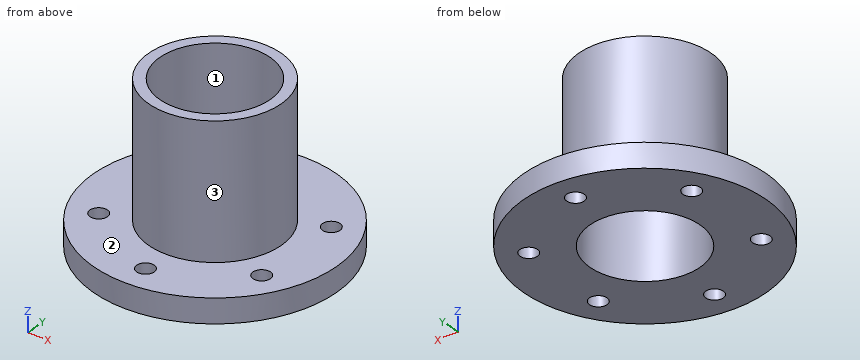
```python
from build123d import *

# Parameters (mm, degrees)
SKETCH1_R               = 110
BOSS_EXTRUDE2_DEPTH     = 22
SKETCH2_R               = 60
BOSS_EXTRUDE3_DEPTH     = 120
CUT_EXTRUDE1_DEPTH      = 211.627633515
CUT_EXTRUDE1_DEPTH_BACK = 211.627633515
SKETCH3_R               = 50
SKETCH4_R               = 8
CUT_EXTRUDE2_DEPTH      = 197.468827044
CIRPATTERN1_COUNT       = 6


with BuildPart() as part:
    # Sketch1 → Boss-Extrude2 (new body)
    with BuildSketch(Plane.XY):
        Circle(SKETCH1_R)
    extrude(amount=BOSS_EXTRUDE2_DEPTH)

    # Sketch2 → Boss-Extrude3 (add)
    with BuildSketch(Plane.XY.offset(22)):
        Circle(SKETCH2_R)
    extrude(amount=BOSS_EXTRUDE3_DEPTH)

    # Sketch3 → Cut-Extrude1 (cut, two sides: drawn at the far end of the back side and taken through both)
    with BuildSketch(Plane.XY.offset(142).offset(-CUT_EXTRUDE1_DEPTH_BACK)):
        Circle(SKETCH3_R)
    extrude(amount=CUT_EXTRUDE1_DEPTH + CUT_EXTRUDE1_DEPTH_BACK, mode=Mode.SUBTRACT)

    # Sketch4 → Cut-Extrude2 (cut, symmetric)
    with BuildSketch(Plane.XY.offset(22)):
        with Locations((0, 85)):
            Circle(SKETCH4_R)
    cut_extrude2 = extrude(amount=CUT_EXTRUDE2_DEPTH, both=True, mode=Mode.SUBTRACT)

    # CirPattern1: Cut-Extrude2 ×6 about axis
    cirpattern1_axis = Axis((0, 0, 0), (0, 0, 1))
    for i in range(1, CIRPATTERN1_COUNT):
        add(cut_extrude2.rotate(cirpattern1_axis, i * 360 / CIRPATTERN1_COUNT), mode=Mode.SUBTRACT)


solid = part.part
```
Source: CAD feature listing. Evaluate the final solid. Frame: model axes, mm. Face numbers are marked on the shaded views. Round coordinates to 2 decimals unless told otherwise and drop trailing zeros. Write each loop counter-clockwise with the first axis right and the second up, starting at its lowest first coordinate (ties: lowest second). Pieces come first, ordered by that corner, then holes. Notation, with made-up numbers: M 17,71 L 47,71 A22 cw 47,80 Z; hole C -1.5,66.5 d9. An arc over 180 degrees is marked long. Answer as a JSON object with one key per item and string values. Group by question number.
(1) Section query A-A on y = 0. Output: boundary loops of the cut face in (x, z), then the cut area to 3 significant figures.
(2) Section query D-D on z = 29. Output: boundary loops of the cut face in (x, y).
(3) Ray query, line 1 (Y direction, x = 0, z = 7.5); line 2 (Z direction, x = -95.5, y = 3); line 3 (X direction, y = 42, z = 12). Return the intervals inside material, ascending. Write a range as [from, to].
(4) First-contact query: pin 1 (1 mm diameter, centred on y = -32.5, z = 41, fed in from +X); pin 2 (18.5 mm diameter, centred on x = 0, y = -85, fed in from +Z); pin 3 (3 mm diameter, centred on y = 23.5, z = 93, fed in from -X). Flat tips, straight axial feed; report the tip coordinate or a pass-through.
(5) Mould query, pull axis Y, two halves, no side actions, for the marked faces 1, 2 and 3. Classes: +Y half, -Y half, draft (parallel to the pull), parting line (faces both ways), or undercut.
(6) Section query B-B on x = 0. Output: boundary loops of the cut face in (y, z).
(7) Section query C-C on y = -42.5. Output: boundary loops of the cut face in (x, z), then the cut area to 3 significant figures.
Computed values:
{
 "1": {"outline": "M -110,0 L -50,0 L -50,142 L -60,142 L -60,22 L -110,22 Z; M 50,0 L 110,0 L 110,22 L 60,22 L 60,142 L 50,142 Z", "area": "5,040 mm^2"},
 "2": {"outline": "C 0,0 d120; hole C 0,0 d100"},
 "3": {"line 1": "[-110, -93], [-77, -50], [50, 77], [93, 110]", "line 2": "[0, 22]", "line 3": "[-101.67, -81.6], [-65.63, -27.13], [27.13, 65.63], [81.6, 101.67]"},
 "4": {"pin 1": "x = 50.75", "pin 2": "z = 22", "pin 3": "x = -55.82"},
 "5": {"face 1": "undercut", "face 2": "draft", "face 3": "parting line"},
 "6": {"outline": "M -110,0 L -93,0 L -93,22 L -110,22 Z; M -77,0 L -50,0 L -50,142 L -60,142 L -60,22 L -77,22 Z; M 50,0 L 77,0 L 77,22 L 60,22 L 60,142 L 50,142 Z; M 93,0 L 110,0 L 110,22 L 93,22 Z"},
 "7": {"outline": "M -101.46,0 L -81.61,0 L -81.61,22 L -101.46,22 Z; M -65.61,0 L -26.34,0 L -26.34,142 L -42.35,142 L -42.35,22 L -65.61,22 Z; M 26.34,0 L 65.61,0 L 65.61,22 L 42.35,22 L 42.35,142 L 26.34,142 Z; M 81.61,0 L 101.46,0 L 101.46,22 L 81.61,22 Z", "area": "6,440 mm^2"}
}
